For this review, take the finished solid that the model builds, in its own axes (mm). Coordinates: 2 decimals unless noted, no trailing zeros. Loops run counter-clockwise (first coordinate to the right, second up) from the corner with the lowest first, then second, coordinate; pieces in that order, holes last. Notation, with made-up numbers: (83, 76) -> (129, 76) arc R23 cw to (129, 90) -> close; hole circle Ø9 at (12.25, 64.25). An arc over 180 degrees is marked (long way). Answer in a Markdown table with one row per item.
from build123d import *

# Parameters (mm, degrees)
ESQUISSE1_R        = 11
BOSS_EXTRU_1_DEPTH = 7
CHANFREIN1_SIZE    = 0.5
CHANFREIN2_SIZE    = 1


with BuildPart() as part:
    # Esquisse1 → Boss.-Extru.1 (new body)
    with BuildSketch(Plane(origin=(0, 0, 0), x_dir=(1, 0, 0), z_dir=(0, 1, 0))):
        with BuildLine():
            Line((0, 15), (55, 15))
            ThreePointArc((55, 15), (70, 0), (55, -15))
            Line((55, -15), (0, -15))
            ThreePointArc((0, -15), (-15, 0), (0, 15))
        make_face()
        with Locations(Location((27.5, 0, 0), (0, 0, 270))):  # turned: the seam where the file's is
            Circle(ESQUISSE1_R, mode=Mode.SUBTRACT)
        with Locations(Location((0, 0, 0), (0, 0, 270))):  # turned: the seam where the file's is
            Circle(ESQUISSE1_R, mode=Mode.SUBTRACT)
        with Locations(Location((55, 0, 0), (0, 0, 270))):  # turned: the seam where the file's is
            Circle(ESQUISSE1_R, mode=Mode.SUBTRACT)
    extrude(amount=BOSS_EXTRU_1_DEPTH)

    # Chanfrein1
    chanfrein1_edges = [part.edges().sort_by_distance(p)[0] for p in [
        (27.5, 0, -11),
        (27.5, 7, -11),
        (0, 0, -11),
        (0, 7, -11),
        (55, 0, -11),
        (55, 7, -11),
    ]]
    chamfer(chanfrein1_edges, length=CHANFREIN1_SIZE)

    # Chanfrein2
    chanfrein2_edges = [part.edges().sort_by_distance(p)[0] for p in [
        (70, 7, 0),
        (27.5, 7, -15),
        (-15, 7, 0),
        (27.5, 0, -15),
        (70, 0, 0),
        (27.5, 0, 15),
        (-15, 0, 0),
        (27.5, 7, 15),
    ]]
    chamfer(chanfrein2_edges, length=CHANFREIN2_SIZE)


solid = part.part
Item 1: Take a section at C-C, the plane y = 4.5. State the section outline as (x, z) points.
Worked answers:
| item | result |
|---|---|
| outline | (0, -15) -> (55, -15) arc R15 ccw to (55, 15) -> (0, 15) arc R15 ccw to start; hole circle Ø22 at (0, 0); hole circle Ø22 at (27.5, 0); hole circle Ø22 at (55, 0) |
Item 2: Insertion check: pin 1 (8 mm diameter, centred on x = 3.5, z = -1, fed in from +Y). The pin has a flat end and moves straight along its axis. Give the tip position at first contact, or say it passes through.
Worked answers:
| item | result |
|---|---|
| pin 1 | through |
Item 3: The part is to be moulded in two halves that separate along Z. For faces 1 (the flat face through (37.3, 7, -6.4)), 2 (the cylindrical face through (70, 3, 0)), 3 (the cylindrical face through (-10.74, 3.46, -2.38)), say which applies: +Z half, -Z half, draft (parallel to the pull), parting line (faces both ways), or undercut.
Worked answers:
| item | result |
|---|---|
| face 1 | draft |
| face 2 | parting line |
| face 3 | undercut |
Item 4: Take a section at A-A, the plane x = 27.5. State the section outline as (y, z) points, and give its area (3 significant figures).
Worked answers:
| item | result |
|---|---|
| outline | (0, -14) -> (1, -15) -> (6, -15) -> (7, -14) -> (7, -11.5) -> (6.5, -11) -> (0.5, -11) -> (0, -11.5) -> close; (0, 11.5) -> (0.5, 11) -> (6.5, 11) -> (7, 11.5) -> (7, 14) -> (6, 15) -> (1, 15) -> (0, 14) -> close |
| area | 53.5 mm² |
Item 5: Take a section at B-B, the plane z = 0. Count the separate pieces of the cut face and the enclosed holes in it, and give its area (4 significant figures).
Worked answers:
| item | result |
|---|---|
| separate pieces | 4 |
| enclosed holes | 0 |
| area | 129.5 mm² |
Item 6: For L1, parallel to X at y = 4.45, z = 0; L2, parallel to X at y = 5.25, z = -9.5; L3, parallel to Z at x = 34.5, y = 1.75, list the stretches that pass through material, from the lowest coordinate up.
Worked answers:
| item | result |
|---|---|
| L1 | -15 to -11, 11 to 16.5, 38.5 to 44, 66 to 70 |
| L2 | -11.61 to -5.55, 5.55 to 21.95, 33.05 to 49.45, 60.55 to 66.61 |
| L3 | -15 to -8.49, 8.49 to 15 |
